Build history of the part. All positions in model axes, mm. A direction names the side the tool comes from. Give positions to 0.01 mm unless a question says otherwise; leave off trailing zeros. Write each loop counter-clockwise with the first axis right and the second up, starting at its lowest first coordinate (ties: lowest second). Pieces come first, ordered by that corner, then holes. Notation, with made-up numbers: (83, 35) -> (122, 35) arc R21 ccw to (122, 69) -> close; hole circle Ø6 at (85, 67.5). An arc over 180 degrees is marked (long way). Put each result on its own line as item: value.
from build123d import *

# Parameters (mm, degrees)
F0_W     = 146.05
F0_H     = 438.15
F1_DEPTH = 9.525
F2_W     = 146.05
F2_H     = 19.05
F3_DEPTH = 6.35
F4_W     = 19.05
F4_H     = 876.3
F5_DEPTH = 12.7
F6_W     = 6.35
F6_H     = 876.3
F7_DEPTH = 12.7
F8_W     = 76.2
F8_H     = 101.6
F9_DEPTH = 19.051


with BuildPart() as f1:
    # F0 (on Front) → F1 (new body, symmetric)
    with BuildSketch(Plane.XZ):
        with Locations((-174.8789953259, 219.075)):
            Rectangle(F0_W, F0_H)
        with Locations((-174.8789953259, -219.075)):
            Rectangle(F0_W, F0_H)
    extrude(amount=F1_DEPTH, both=True)

    # F2 (on face) → F3 (cut)
    with BuildSketch(Plane(origin=(0, 9.525, 0), x_dir=(-1, 0, 0), z_dir=(0, 1, 0))):
        with Locations((174.8789953259, 309.5625)):
            Rectangle(F2_W, F2_H)
    extrude(amount=-F3_DEPTH, mode=Mode.SUBTRACT)

    # F4 (on face) → F5 (cut)
    with BuildSketch(Plane.XZ.offset(9.525)):
        with Locations((-111.3789953259, 0)):
            Rectangle(F4_W, F4_H)
    extrude(amount=-F5_DEPTH, mode=Mode.SUBTRACT)

    # F6 (on face) → F7 (cut)
    with BuildSketch(Plane.XZ.offset(9.525)):
        with Locations((-244.7289953259, 0)):
            Rectangle(F6_W, F6_H)
    extrude(amount=-F7_DEPTH, mode=Mode.SUBTRACT)

    # F8 (on face) → F9 (cut, through all)
    with BuildSketch(Plane(origin=(0, 9.525, 0), x_dir=(-1, 0, 0), z_dir=(0, 1, 0))):
        with Locations((209.8039953259, 387.35)):
            Rectangle(F8_W, F8_H)
    extrude(amount=-F9_DEPTH, mode=Mode.SUBTRACT)


solid = f1.part
1) Pin check, flat tips, straight feed: pin 1 (5 mm diameter, centred on x = -211, y = -6, fed in from +Z); pin 2 (5.5 mm diameter, centred on x = -168.5, z = 306.5, fed in from +Y) (3 decimals); pin 3 (1.9 mm diameter, centred on x = -245.5, z = 329, fed in from -Y) (3 decimals). Stop position of each tip, or through.
Filled sheet:
pin 1: z = 336.55
pin 2: y = 3.175
pin 3: y = 3.175
2) Slice it at C-C (z = -97.5). Write the cut outline in (x, y) (3 decimals).
Filled sheet:
outline: (-247.904, 3.175) -> (-241.554, 3.175) -> (-241.554, -9.525) -> (-120.904, -9.525) -> (-120.904, 3.175) -> (-101.854, 3.175) -> (-101.854, 9.525) -> (-247.904, 9.525) -> close
3) Slice it at D-D (z = 348.5). Write the cut outline in (x, y) (3 decimals), plus the area to 3 significant figures.
Filled sheet:
outline: (-171.704, -9.525) -> (-120.904, -9.525) -> (-120.904, 3.175) -> (-101.854, 3.175) -> (-101.854, 9.525) -> (-171.704, 9.525) -> close
area: 1,090 mm2
4) Tool access for faces 1 (the flat face through (-112, 3.175, -64)), 2 (the flat face through (-180, 3.175, 310)), 3 (the flat face through (-176, 9.525, -64)), 4 (the flat face through (-182, -9.525, 6)), 5 (the flat face through (-171.704, 0, 387)): list every direction of +Z, -Z, +X, -X, +Y, -Y with a clear straight run to the whole face (end or side of a thin tool).
Filled sheet:
face 1: +Z, -Z, +X, -Y
face 2: +X, -X, +Y
face 3: +Z, -Z, +X, -X, +Y
face 4: +Z, -Z, +X, -X, -Y
face 5: +Z, -X, +Y, -Y
5) Slice it at A-A (y = 6.25). Write the cut outline in (x, z).
Filled sheet:
outline: (-247.9, -438.15) -> (-101.85, -438.15) -> (-101.85, 300.04) -> (-247.9, 300.04) -> close; (-247.9, 319.09) -> (-101.85, 319.09) -> (-101.85, 438.15) -> (-171.7, 438.15) -> (-171.7, 336.55) -> (-247.9, 336.55) -> close
6) Wall check: L1, parallel to Z at x = -133, y = 5.25; L2, parallel to Z at x = -183.5, y = 6.75; L3, parallel to X at y = -3, z = 203. Give the ranges that are in metal, low to high.
Filled sheet:
L1: -438.15 to 300.04, 319.09 to 438.15
L2: -438.15 to 300.04, 319.09 to 336.55
L3: -241.55 to -120.9
